The drawing under review shows one solid part. Ordinate dimensions are in mm from its lowest x, y, z. Coordinates: 2 decimals unless noted, no trailing zeros. Write each loop counter-clockwise with the first axis right and the second up, starting at its lowest first coordinate (ties: lowest second). Pieces come first, ordered by that corner, then holes. Notation, with made-up numbers: M -6.75,76 L 11.25,76 A17 ccw 11.25,81 Z; hole C 26.5,-0.75 d7. An arc over 180 degrees is marked long. Write item = value, one per line.
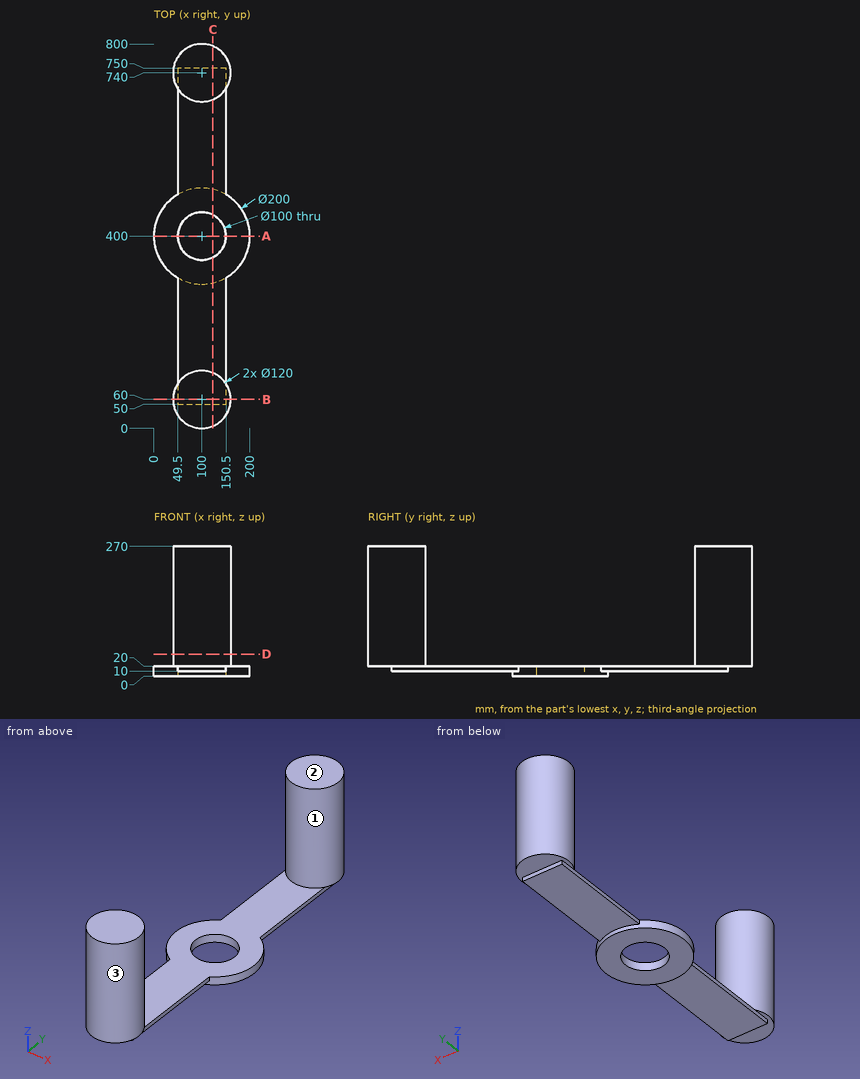
Q1. Consider section C-C, the plane x = 123. State the section outline as (y, z) points, and give its area (3 significant figures).
Check result:
outline = M 4.58,20 L 50,20 L 50,10 L 302.68,10 L 302.68,0 L 355.6,0 L 355.6,20 L 115.42,20 L 115.42,270 L 4.58,270 Z; M 444.4,0 L 497.32,0 L 497.32,10 L 750,10 L 750,20 L 795.42,20 L 795.42,270 L 684.58,270 L 684.58,20 L 444.4,20 Z
area = 62,600 mm²
Q2. Consider section B-B, the plane y = 60. State the section outline as (x, z) points, and give its area (3 significant figures).
Check result:
outline = M 40,20 L 49.5,20 L 49.5,10 L 150.5,10 L 150.5,20 L 160,20 L 160,270 L 40,270 Z
area = 31,000 mm²
Q3. Wall thickness on line 1 (Y direction, x = 100, z = 6.25); line 2 (X direction, y = 400, z = 14); line 3 (Z direction, x = 142, y = 44): over which ranges is each line inside the solid? List them lowest first.
Check result:
line_1 = 300 to 350, 450 to 500
line_2 = 0 to 50, 150 to 200
line_3 = 20 to 270
Q4. Consider section D-D, the plane z = 45.5. State the section outline as (x, y) points, and give its area (3 significant figures).
Check result:
outline = C 100,60 d120; C 100,740 d120
area = 22,600 mm²
Q5. Consider section A-A, the plane y = 400. State the section outline as (x, z) points.
Check result:
outline = M 0,0 L 50,0 L 50,20 L 0,20 Z; M 150,0 L 200,0 L 200,20 L 150,20 Z
Q6. For P1, Ø3, axis at y = 136.5, z = 16.5, coming from the -X side; P2, Ø8, axis at x = 76.5, z = 13, coming from the +Y side; P3, Ø1, axis at x = 129, y = 146.5, coming from the -Z side, all flat-tipped, find the tip position at first contact; note any pin that passes through.
Check result:
P1 = 49.5
P2 = 750
P3 = 10
Q7. The part is to be moulded in two halves that separate along Y. For the marked faces 1, 2 and 3, say which applies: +Y half, -Y half, draft (parallel to the pull), parting line (faces both ways), or undercut.
Check result:
face_1 = undercut
face_2 = draft
face_3 = undercut
